Answer from the drawing. Dimensions are ordinates in mm from the lowest x, y and z of the part. A direction names the side the tool comes from. Coordinates: 2 decimals unless noted, no trailing zeros. Order: outer loops, then holes, each group sorted by start corner. A loop starts at its lowest first (then second) coordinate and runs counter-clockwise, first axis right, second up.
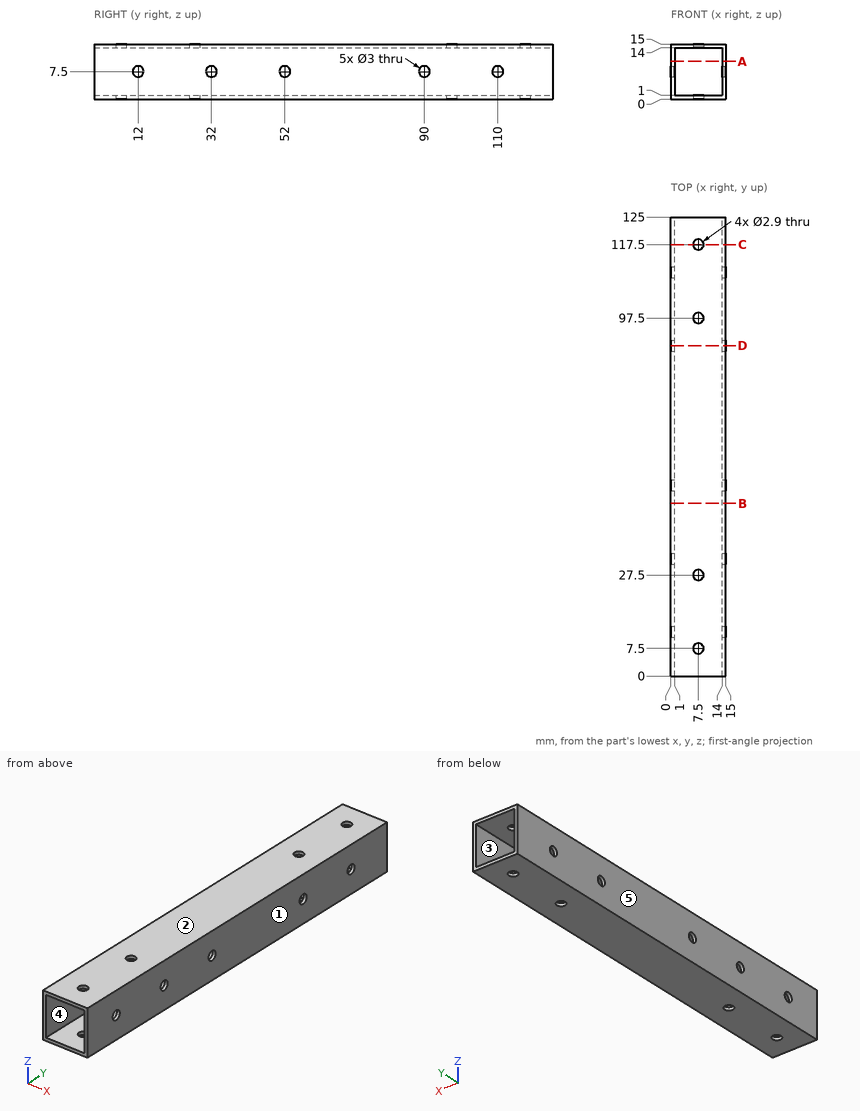
1. The mould has two halves that part along Z. Classify the marked faces 1, 2 and 3: released by +Z, released by -Z, zero draft, split by the parting line, or undercut.
2. The part is cut by section A-A (z = 10.25). Determine the outline of the cut face in (x, y).
3. Consider probe 1 along Y at (x, z) = (7.5, 14.7); probe 2 along Y at (x, z) = (14.25, 7.5); probe 3 along Z at (x, y) = (14.75, 110). Determine where each line is inside the solid, lowest interval first.
4. The part is cut by section B-B (y = 47). Determine the outline of the cut face in (x, z), plus the area to 3 significant figures.
5. The part is cut by section D-D (y = 90). Determine the outline of the cut face in (x, z), plus the area to 3 significant figures.
6. For the marked faces 4 and 5, determine the directions among +Z, -Z, +X, -X, +Y, -Y from which every point of the face is accessible in a straight line to the end or side of a thin tool.
7. The part is cut by section C-C (y = 117.5). Determine the outline of the cut face in (x, z), plus the area to 3 significant figures.
Worked out:
1. face 1: zero draft
1. face 2: released by +Z
1. face 3: undercut
2. outline: (0, 0) - (1, 0) - (1, 125) - (0, 125) - close; (14, 0) - (15, 0) - (15, 125) - (14, 125) - close
3. probe 1: y = 0 to 6.05, 8.95 to 26.05, 28.95 to 96.05, 98.95 to 116.05, 118.95 to 125
3. probe 2: y = 0 to 10.5, 13.5 to 30.5, 33.5 to 50.5, 53.5 to 88.5, 91.5 to 108.5, 111.5 to 125
3. probe 3: z = 0 to 6, 9 to 15
4. outline: (0, 0) - (15, 0) - (15, 15) - (0, 15) - close; hole (1, 1) - (14, 1) - (14, 14) - (1, 14) - close
4. area: 56.0 mm2
5. outline: (0, 0) - (15, 0) - (15, 6) - (14, 6) - (14, 1) - (1, 1) - (1, 6) - (0, 6) - close; (0, 9) - (1, 9) - (1, 14) - (14, 14) - (14, 9) - (15, 9) - (15, 15) - (0, 15) - close
5. area: 50.0 mm2
6. face 4: +Y, -Y
6. face 5: +Z, -Z, -X, +Y, -Y
7. outline: (0, 0) - (6.05, 0) - (6.05, 1) - (1, 1) - (1, 14) - (6.05, 14) - (6.05, 15) - (0, 15) - close; (8.95, 0) - (15, 0) - (15, 15) - (8.95, 15) - (8.95, 14) - (14, 14) - (14, 1) - (8.95, 1) - close
7. area: 50.2 mm2
